from build123d import *

# Parameters (mm, degrees)
EXTRUDE_2_DEPTH     = 60
SKETCH_4_R          = 1.7
CUT_EXTRUDE_1_DEPTH = 131.862523283
SKETCH_5_R          = 1.7
CUT_EXTRUDE_2_DEPTH = 131.862523283
SKETCH_6_R          = 2.65
EXTRUDE_4_DEPTH     = 5
RIB_1_REACH         = 110.467
RIB_4_REACH         = 110.467
SKETCH_13_WALL_W    = 247.21744068
SKETCH_13_WALL_H    = 35


with BuildPart() as part:
    # 草图3 → 凸台-拉伸2 (new body)
    with BuildSketch(Plane(origin=(0, 0, 0), x_dir=(1, 0, 0), z_dir=(0, 1, 0))):
        Polygon((54, 54), (49, 54), (49, -49), (-54, -49), (-54, -54), (54, -54), align=None)
    extrude(amount=EXTRUDE_2_DEPTH)

    # 草图4 → 切除-拉伸1 (cut, through all)
    with BuildSketch(Plane(origin=(0, 0, 49), x_dir=(-1, 0, 0), z_dir=(0, 0, -1))):
        with Locations((36.5, 37.5)):
            Circle(SKETCH_4_R)
        with Locations(Location((36.5, 12.5, 0), (0, 0, 180))):
            Circle(SKETCH_4_R)
        with Locations((11.5, 12.5)):
            Circle(SKETCH_4_R)
        with Locations(Location((11.5, 37.5, 0), (0, 0, 180))):
            Circle(SKETCH_4_R)
    extrude(amount=-CUT_EXTRUDE_1_DEPTH, mode=Mode.SUBTRACT)

    # 草图5 → 切除-拉伸2 (cut, through all)
    with BuildSketch(Plane.ZY.offset(-49)):
        with Locations((-36.5, 37.5)):
            Circle(SKETCH_5_R)
        with Locations(Location((-36.5, 12.5, 0), (0, 0, 180))):
            Circle(SKETCH_5_R)
        with Locations((-11.5, 12.5)):
            Circle(SKETCH_5_R)
        with Locations(Location((-11.5, 37.5, 0), (0, 0, 180))):
            Circle(SKETCH_5_R)
    extrude(amount=-CUT_EXTRUDE_2_DEPTH, mode=Mode.SUBTRACT)

    # 草图6 → 凸台-拉伸4 (add)
    with BuildSketch(Plane(origin=(0, 60, 0), x_dir=(1, 0, 0), z_dir=(0, 1, 0))):
        Polygon((-54, -49), (-54, -54), (54, -54), (54, 54), (49, 54), (11.642135624, -11.642135624), align=None)
        with Locations(Location((1.742640687, -35.683766184, 0), (0, 0, 270))):
            Circle(SKETCH_6_R, mode=Mode.SUBTRACT)
        with Locations(Location((35.683766184, -1.742640687, 0), (0, 0, 90))):
            Circle(SKETCH_6_R, mode=Mode.SUBTRACT)
        with Locations(Location((18.713203436, -18.713203436, 0), (0, 0, 270))):
            Circle(SKETCH_6_R, mode=Mode.SUBTRACT)
    extrude(amount=EXTRUDE_4_DEPTH)

    # 草图10 walls → 筋1 (add, up to next)
    with BuildSketch(Plane(origin=(0, 0, 14), x_dir=(-1, 0, 0), z_dir=(0, 0, -1)), mode=Mode.PRIVATE) as rib_1_sk1:
        Polygon((18.817089986, 163.891167178), (-149.296374034, -16.112124581), (-123.717265916, -40.00164588), (44.396198104, 140.00164588), align=None)
    rib_1_tool1 = extrude(rib_1_sk1.sketch, amount=-RIB_1_REACH, mode=Mode.PRIVATE) - part.part
    add(rib_1_tool1.solids().sort_by_distance((39.660533906, 50, 14))[0])

    # 草图13 wall → 筋4 (add, up to next)
    with BuildSketch(Plane(origin=(14, 50, 39), x_dir=(0, -0.707106781187, 0.707106781187), z_dir=(0, 0.707106781187, 0.707106781187)), mode=Mode.PRIVATE) as rib_4_sk1:
        with Locations((0, 17.5)):
            Rectangle(SKETCH_13_WALL_W, SKETCH_13_WALL_H)
    rib_4_tool1 = extrude(rib_4_sk1.sketch, amount=RIB_4_REACH, mode=Mode.PRIVATE) - part.part
    add(rib_4_tool1.solids().sort_by_distance((14, 50, 39))[0])


solid = part.part
Geometry: final body of the model. Coordinates: model frame, mm. A direction names the side the tool comes from. Give positions to 0.01 mm unless a question says otherwise; leave off trailing zeros. Write each loop counter-clockwise with the first axis right and the second up, starting at its lowest first coordinate (ties: lowest second). Pieces come first, ordered by that corner, then holes.
(1) Cut plane B-B, the plane x = -11.5. Return loops of the section in (y, z).
(2) Cut plane A-A, the plane y = 12.5. Return loops of the section in (x, z).
(3) Cut plane C-C, the plane z = -11.5. Return loops of the section in (x, y).
(4) Ray query, line 1 (Y direction, x = 51.5, z = -11.5); line 2 (X direction, y = 45.5, z = -44); line 3 (X direction, y = 12, z = 50). Return the intervals inside material, ascending.
(5) First-contact query: P1, Ø4, axis at x = 18.71, z = 18.71, coming from the +Y side; P2, Ø4.5, axis at x = -36.5, y = 12.5, coming from the -Z side; P3, Ø10, axis at x = 23.5, z = -0.5, coming from the -Y side; P4, Ø4.5, axis at y = 12.5, z = -36.5, coming from the -X side. Flat tips, straight axial feed; report the tip coordinate or a pass-through.
(6) Mould query, pull axis Z, two halves, no side actions, for faces 1 (the flat face through (13, 60, 16)), 2 (the cylindrical face through (34.888, 62.465, -0.785)), 3 (the cylindrical face through (51.5, 39, -12.3)), 4 (the flat face through (30.583, 62.465, -21.638)). Classes: released by +Z, released by -Z, zero draft, split by the parting line, or undercut.
(7) Cut plane D-D, the plane y = 28. Return loops of the section in (x, z).
(8) Access query for faces 5 (the flat face through (42, 52, 14)), 6 (the flat face through (54, 32, 1)). Directions: +Z, -Z, +X, -X, +Y, -Y. A direction counts if a zero-diameter tool reaches every point of the face in a straight line with its end or side. Return the directions, or none.
Values follow:
1. outline: (0, 49) - (10.8, 49) - (10.8, 54) - (0, 54) - close; (14.2, 49) - (35.8, 49) - (35.8, 54) - (14.2, 54) - close; (39.2, 49) - (60, 49) - (60, 24.81) - (65, 24.81) - (65, 54) - (39.2, 54) - close
2. outline: (-54, 49) - (-38.2, 49) - (-38.2, 54) - (-54, 54) - close; (-34.8, 49) - (-13.2, 49) - (-13.2, 54) - (-34.8, 54) - close; (-9.8, 49) - (49, 49) - (49, -9.8) - (54, -9.8) - (54, 54) - (-9.8, 54) - close; (49, -54) - (54, -54) - (54, -38.2) - (49, -38.2) - close; (49, -34.8) - (54, -34.8) - (54, -13.2) - (49, -13.2) - close
3. outline: (24.81, 60) - (49, 60) - (49, 39.2) - (54, 39.2) - (54, 65) - (24.81, 65) - close; (49, 0) - (54, 0) - (54, 10.8) - (49, 10.8) - close; (49, 14.2) - (54, 14.2) - (54, 35.8) - (49, 35.8) - close
4. line 1: y = 0 to 10.8, 14.2 to 35.8, 39.2 to 65
4. line 2: x = 49 to 54
4. line 3: x = -54 to -38.12, -34.88 to -13.12, -9.88 to 54
5. P1: passes through
5. P2: stops at z = 49
5. P3: stops at y = 60
5. P4: stops at x = 49
6. face 1: zero draft
6. face 2: undercut
6. face 3: undercut
6. face 4: released by -Z
7. outline: (-54, 49) - (49, 49) - (49, -54) - (54, -54) - (54, 54) - (-54, 54) - close
8. face 5: -Z, -X, -Y
8. face 6: +Z, -Z, +X, +Y, -Y
